Drawing for the job (mm, zero at the part's lowest x, y, z). A direction names the side the tool comes from. Coordinates: 2 decimals unless noted, no trailing zeros. Loops run counter-clockwise (first coordinate to the right, second up) from the corner with the lowest first, then second, coordinate; pieces in that order, holes last. Notation, with made-up numbers: (-38.5, 39) -> (-3.5, 39) arc R15 ccw to (-3.5, 58) -> close; hole circle Ø11 at (-35, 20). An arc over 180 degrees is marked (long way). Write each question's results on one line, items separated by ' | '.
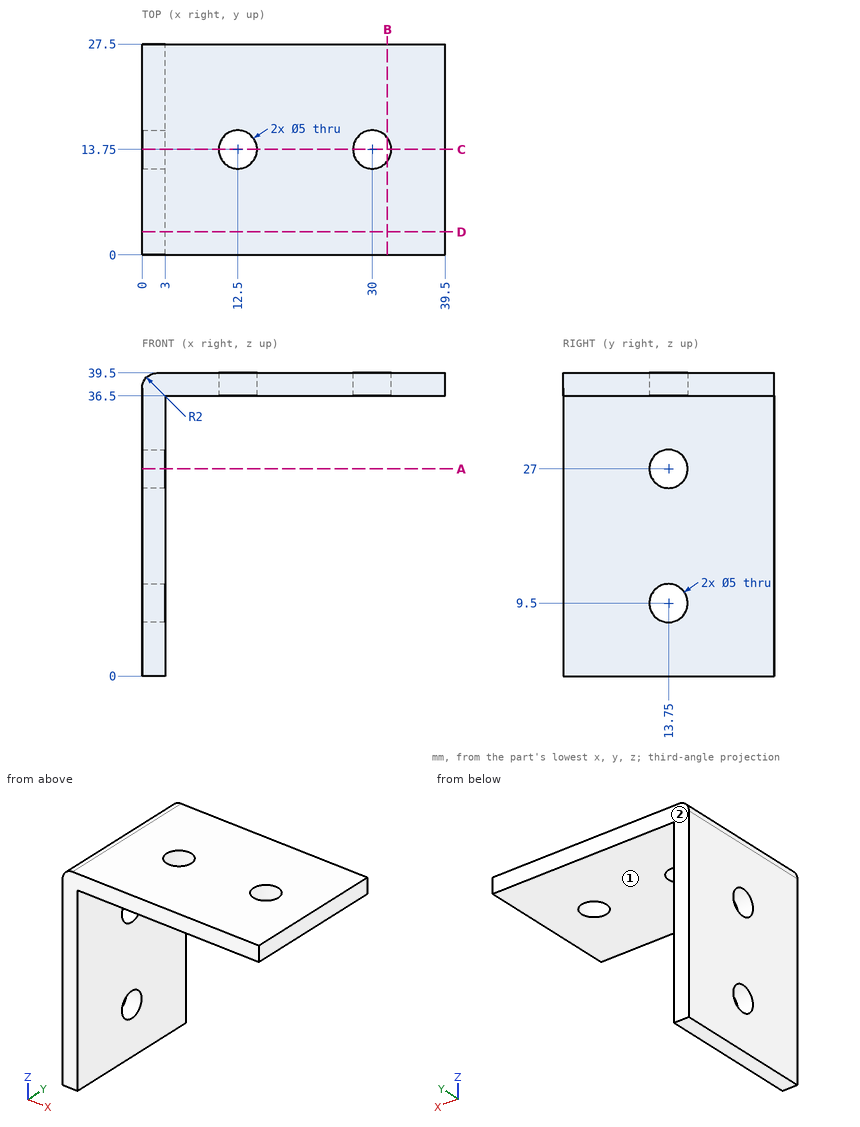
1) Slice it at C-C (y = 13.75). Write the cut outline in (x, z), then the cut area to 3 significant figures.
Outcome:
outline: (0, 0) -> (3, 0) -> (3, 7) -> (0, 7) -> close; (0, 12) -> (3, 12) -> (3, 24.5) -> (0, 24.5) -> close; (0, 29.5) -> (3, 29.5) -> (3, 36.5) -> (10, 36.5) -> (10, 39.5) -> (2, 39.5) arc R2 ccw to (0, 37.5) -> close; (15, 36.5) -> (27.5, 36.5) -> (27.5, 39.5) -> (15, 39.5) -> close; (32.5, 36.5) -> (39.5, 36.5) -> (39.5, 39.5) -> (32.5, 39.5) -> close | area: 167 mm^2
2) Slice it at D-D (y = 3). Write the cut outline in (x, z), then the cut area to 3 significant figures.
Outcome:
outline: (0, 0) -> (3, 0) -> (3, 36.5) -> (39.5, 36.5) -> (39.5, 39.5) -> (2, 39.5) arc R2 ccw to (0, 37.5) -> close | area: 227 mm^2
3) Slice it at B-B (x = 32). Write the cut outline in (y, z), then the cut area to 3 significant figures.
Outcome:
outline: (0, 36.5) -> (12.25, 36.5) -> (12.25, 39.5) -> (0, 39.5) -> close; (15.25, 36.5) -> (27.5, 36.5) -> (27.5, 39.5) -> (15.25, 39.5) -> close | area: 73.5 mm^2
4) Pin check, flat tips, straight feed: pin 1 (1.5 mm diameter, centred on y = 12, z = 25, fed in from +X); pin 2 (3 mm diameter, centred on y = 13.75, z = 9.5, fed in from -X); pin 3 (3 mm diameter, centred on x = 23.5, y = 19, fed in from -Z). Stop position of each tip, or through.
Outcome:
pin 1: stops at x = 3 | pin 2: passes through | pin 3: stops at z = 36.5
5) Slice it at A-A (z = 27). Write the cut outline in (x, y), then the cut area to 3 significant figures.
Outcome:
outline: (0, 0) -> (3, 0) -> (3, 11.25) -> (0, 11.25) -> close; (0, 16.25) -> (3, 16.25) -> (3, 27.5) -> (0, 27.5) -> close | area: 67.5 mm^2
6) Which spindle directions (+Z, -Z, +X, -X, +Y, -Y) get a long thin tool onto all of the face, cutting with end or side? Do the marked faces 1 and 2. Say none if no direction does.
Outcome:
face 1: -Z, +X, +Y, -Y | face 2: +Z, -Z, +X, -X, +Y
7) Drill centre lines: L1, parallel to Y at x = 1.5, z = 9.5; L2, parallel to X at y = 13.75, z = 35.5; L3, parallel to Z at x = 12, y = 8.5. Where is each one in solid material? Low to high. Write a range as from..to.
Outcome:
L1: y = 0..11.25, 16.25..27.5 | L2: x = 0..3 | L3: z = 36.5..39.5
